Read the model definition and answer for the solid it produces. Units are mm, in the model's axes. A direction names the side the tool comes from. Round coordinates to 2 decimals unless told otherwise and drop trailing zeros. Order: outer loops, then holes, each group sorted by start corner. A loop starts at its lowest first (then second) coordinate and runs counter-clockwise, first axis right, second up. Notation, with made-up numbers: M -16.5,3 L 21.5,3 A27 ccw 21.5,30 Z; hole C 18,56 d2. An arc over 180 degrees is marked long. Answer as CSV lines item,"result".
```python
from build123d import *

# Parameters (mm, degrees)
F1_DEPTH = 8


with BuildPart() as f1:
    # F0 (on Top) → F1 (new body)
    with BuildSketch(Plane.XY):
        with BuildLine():
            Line((287.5, 150), (-287.5, 150))
            Line((-287.5, 150), (-641.464466, 503.964466))
            ThreePointArc((-641.464466, 503.964466), (-646.913417, 505.04833), (-650, 500.428932))
            Line((-650, 500.428932), (-650, 220.784271))
            ThreePointArc((-650, 220.784271), (-648.477591, 213.130603), (-644.142136, 206.642136))
            Line((-644.142136, 206.642136), (-293.357864, -144.142136))
            ThreePointArc((-293.357864, -144.142136), (-286.869397, -148.477591), (-279.215729, -150))
            Line((-279.215729, -150), (279.215729, -150))
            ThreePointArc((279.215729, -150), (286.869397, -148.477591), (293.357864, -144.142136))
            Line((293.357864, -144.142136), (644.142136, 206.642136))
            ThreePointArc((644.142136, 206.642136), (648.477591, 213.130603), (650, 220.784271))
            Line((650, 220.784271), (650, 500.428932))
            ThreePointArc((650, 500.428932), (646.913417, 505.04833), (641.464466, 503.964466))
            Line((641.464466, 503.964466), (287.5, 150))
        make_face()
    extrude(amount=F1_DEPTH)


solid = f1.part
```
Item 1: A tool of negligible diameter and unlimited length cuts with its end or side. For faces 1 (the face through (-462, 324.5, 3.9)), 2 (the face through (-9, 109, 0)), from which of +Z, -Z, +X, -X, +Y, -Y can it reach the whole face along a straight path? Write none if from no direction.
Ans:
face 1,"+Z, -Z, +Y"
face 2,"-Z, +X, -X, +Y, -Y"
Item 2: A cutting plane is placed at C-C, the plane y = 261. Determine the outline of the cut face in (x, z), and give its area (3 significant figures).
Ans:
outline,"M -650,0 L -398.5,0 L -398.5,8 L -650,8 Z; M 398.5,0 L 650,0 L 650,8 L 398.5,8 Z"
area,"4,020 mm2"
Item 3: A cutting plane is placed at B-B, the plane z = 2.5. Determine the outline of the cut face in (x, y).
Ans:
outline,"M -650,220.78 A20 ccw -644.14,206.64 L -293.36,-144.14 A20 ccw -279.22,-150 L 279.22,-150 A20 ccw 293.36,-144.14 L 644.14,206.64 A20 ccw 650,220.78 L 650,500.43 A5 ccw 641.46,503.96 L 287.5,150 L -287.5,150 L -641.46,503.96 A5 ccw -650,500.43 Z"
Item 4: A cutting plane is placed at D-D, the plane x = 171.5. Determine the outline of the cut face in (y, z).
Ans:
outline,"M -150,0 L 150,0 L 150,8 L -150,8 Z"
Item 5: A cutting plane is placed at A-A, the plane y = 328. Determine the outline of the cut face in (x, z), and give its area (3 significant figures).
Ans:
outline,"M -650,0 L -465.5,0 L -465.5,8 L -650,8 Z; M 465.5,0 L 650,0 L 650,8 L 465.5,8 Z"
area,"2,950 mm2"
Item 6: Determine the mould class of faces 3 (the face through (466.3, 28.8, 3.9)), 4 (the face through (-9, 109, 8)), 5 (the face through (467, 329.5, 3.9)), 6 (the face through (-471.2, 33.7, 3.9)) for opening direction X: +X half, -X half, draft (parallel to the pull), parting line (faces both ways), or undercut.
Ans:
face 3,"+X half"
face 4,"draft"
face 5,"undercut"
face 6,"-X half"
Item 7: Flat-ended cylindrical pins translate along their axes: pin 1 (4 mm diameter, centred on y = -21.5, z = 4.5, fed in from -X); pin 2 (3 mm diameter, centred on y = -61, z = 7, fed in from +X). Find the tip coordinate at first contact, or state that the pin passes through.
Ans:
pin 1,"x = -418"
pin 2,"x = 378"
Item 8: Find the intervals of material crossed by probe 1 along Y at (x, z) = (-182.5, 4.5); probe 2 along X at (y, z) = (193, 6.25); probe 3 along X at (y, z) = (228, 4.75), in increasing order. Write a range as [from, to].
Ans:
probe 1,"[-150, 150]"
probe 2,"[-630.5, -330.5], [330.5, 630.5]"
probe 3,"[-650, -365.5], [365.5, 650]"
